from build123d import *

# Parameters (mm, degrees)
F0_R     = 1.5875
F1_DEPTH = 19.05
F0_R_2   = 3.175
F2_DEPTH = 6.35
F3_R     = 1.27


with BuildPart() as f1:
    # F0 (on Top) → F1 (new body)
    with BuildSketch(Plane.XY):
        with BuildLine():
            ThreePointArc((82.8215071839, 56.5294814298), (0, 37.38), (-82.8215071839, 56.5294814298))
            ThreePointArc((-82.8215071839, 56.5294814298), (-92.8246316261, 54.4975844509), (-93.4439756283, 44.3089870526))
            ThreePointArc((-93.4439756283, 44.3089870526), (-79.88, 0), (-93.4439756283, -44.3089870526))
            ThreePointArc((-93.4439756283, -44.3089870526), (-92.8246316261, -54.4975844509), (-82.8215071839, -56.5294814298))
            ThreePointArc((-82.8215071839, -56.5294814298), (0, -37.38), (82.8215071839, -56.5294814298))
            ThreePointArc((82.8215071839, -56.5294814298), (92.8246316261, -54.4975844509), (93.4439756283, -44.3089870526))
            ThreePointArc((93.4439756283, -44.3089870526), (79.88, 0), (93.4439756283, 44.3089870526))
            ThreePointArc((93.4439756283, 44.3089870526), (92.8246316261, 54.4975844509), (82.8215071839, 56.5294814298))
        make_face()
        with Locations((-86.5, -49)):
            Circle(F0_R, mode=Mode.SUBTRACT)
        with BuildLine():
            ThreePointArc((-44.7490329893, -12.754), (-43.0382407412, -13.2414304642), (-41.8412453259, -14.557333405))
            ThreePointArc((-41.8412453259, -14.557333405), (-39.2272080278, -18.9335940639), (-35.965811948, -22.8512647956))
            ThreePointArc((-35.965811948, -22.8512647956), (-35.1953196756, -26.0911928639), (-37.6837042763, -28.304501317))
            ThreePointArc((-37.6837042763, -28.304501317), (-53.5961461859, -32.0117479156), (-69.1555424288, -36.9971940769))
            ThreePointArc((-69.1555424288, -36.9971940769), (-72.5826288572, -36.2271539786), (-73.3024493232, -32.7891688656))
            ThreePointArc((-73.3024493232, -32.7891688656), (-70.5039949655, -24.2377869494), (-68.556245082, -15.4534970032))
            ThreePointArc((-68.556245082, -15.4534970032), (-67.4497325668, -13.5190259244), (-65.356580963, -12.754))
            Line((-65.356580963, -12.754), (-44.7490329893, -12.754))
        make_face(mode=Mode.SUBTRACT)
        with Locations((86.5, -49)):
            Circle(F0_R, mode=Mode.SUBTRACT)
        with BuildLine():
            ThreePointArc((-12.5, -12.5), (-25, 0), (-12.5, 12.5))
            Line((-12.5, 12.5), (12.5, 12.5))
            ThreePointArc((12.5, 12.5), (25, 0), (12.5, -12.5))
            Line((12.5, -12.5), (-12.5, -12.5))
        make_face(mode=Mode.SUBTRACT)
        with BuildLine():
            ThreePointArc((65.356580963, -12.754), (67.4497325668, -13.5190259244), (68.556245082, -15.4534970032))
            ThreePointArc((68.556245082, -15.4534970032), (70.5039949655, -24.2377869494), (73.3024493232, -32.7891688656))
            ThreePointArc((73.3024493232, -32.7891688656), (72.5826288572, -36.2271539786), (69.1555424288, -36.9971940769))
            ThreePointArc((69.1555424288, -36.9971940769), (53.5961461859, -32.0117479156), (37.6837042763, -28.304501317))
            ThreePointArc((37.6837042763, -28.304501317), (35.1953196756, -26.0911928639), (35.965811948, -22.8512647956))
            ThreePointArc((35.965811948, -22.8512647956), (39.2272080278, -18.9335940639), (41.8412453259, -14.557333405))
            ThreePointArc((41.8412453259, -14.557333405), (43.0382407412, -13.2414304642), (44.7490329893, -12.754))
            Line((44.7490329893, -12.754), (65.356580963, -12.754))
        make_face(mode=Mode.SUBTRACT)
        with BuildLine():
            ThreePointArc((-73.3024493232, 32.7891688656), (-72.5826288572, 36.2271539786), (-69.1555424288, 36.9971940769))
            ThreePointArc((-69.1555424288, 36.9971940769), (-53.5961461859, 32.0117479156), (-37.6837042763, 28.304501317))
            ThreePointArc((-37.6837042763, 28.304501317), (-35.1953196756, 26.0911928639), (-35.965811948, 22.8512647956))
            ThreePointArc((-35.965811948, 22.8512647956), (-39.2272080278, 18.9335940639), (-41.8412453259, 14.557333405))
            ThreePointArc((-41.8412453259, 14.557333405), (-43.0382407412, 13.2414304642), (-44.7490329893, 12.754))
            Line((-44.7490329893, 12.754), (-65.356580963, 12.754))
            ThreePointArc((-65.356580963, 12.754), (-67.4497325668, 13.5190259244), (-68.556245082, 15.4534970032))
            ThreePointArc((-68.556245082, 15.4534970032), (-70.5039949655, 24.2377869494), (-73.3024493232, 32.7891688656))
        make_face(mode=Mode.SUBTRACT)
        with Locations((-86.5, 49)):
            Circle(F0_R, mode=Mode.SUBTRACT)
        with BuildLine():
            ThreePointArc((35.965811948, 22.8512647956), (35.1953196756, 26.0911928639), (37.6837042763, 28.304501317))
            ThreePointArc((37.6837042763, 28.304501317), (53.5961461859, 32.0117479156), (69.1555424288, 36.9971940769))
            ThreePointArc((69.1555424288, 36.9971940769), (72.5826288572, 36.2271539786), (73.3024493232, 32.7891688656))
            ThreePointArc((73.3024493232, 32.7891688656), (70.5039949655, 24.2377869494), (68.556245082, 15.4534970032))
            ThreePointArc((68.556245082, 15.4534970032), (67.4497325668, 13.5190259244), (65.356580963, 12.754))
            Line((65.356580963, 12.754), (44.7490329893, 12.754))
            ThreePointArc((44.7490329893, 12.754), (43.0382407412, 13.2414304642), (41.8412453259, 14.557333405))
            ThreePointArc((41.8412453259, 14.557333405), (39.2272080278, 18.9335940639), (35.965811948, 22.8512647956))
        make_face(mode=Mode.SUBTRACT)
        with Locations((86.5, 49)):
            Circle(F0_R, mode=Mode.SUBTRACT)
    extrude(amount=F1_DEPTH)

    # F0 (on Top) → F2 (cut)
    with BuildSketch(Plane.XY):
        with BuildLine():
            Line((12.5, 12.5), (-12.5, 12.5))
            ThreePointArc((-12.5, 12.5), (-25, 0), (-12.5, -12.5))
            Line((-12.5, -12.5), (12.5, -12.5))
            ThreePointArc((12.5, -12.5), (25, 0), (12.5, 12.5))
        make_face()
        with Locations((-12.5, 0)):
            Circle(F0_R_2, mode=Mode.SUBTRACT)
        with Locations((12.5, 0)):
            Circle(F0_R_2, mode=Mode.SUBTRACT)
    extrude(amount=F2_DEPTH, mode=Mode.SUBTRACT)

    # F3
    f3_edges = [f1.edges().sort_by_distance(p)[0] for p in [
        (-79.88, 0, 19.05),
        (-92.824632, -54.497584, 19.05),
        (0, -37.38, 19.05),
        (92.824632, -54.497584, 19.05),
        (79.88, 0, 19.05),
        (92.824632, 54.497584, 19.05),
        (0, 37.38, 19.05),
        (-92.824632, 54.497584, 19.05),
    ]]
    fillet(f3_edges, radius=F3_R)


solid = f1.part
Here's how the part is built. I have some questions about the finished solid (model axes, mm). A direction names the side the tool comes from. Coordinates: 2 decimals unless noted, no trailing zeros. Write each loop counter-clockwise with the first axis right and the second up, starting at its lowest first coordinate (ties: lowest second). Pieces come first, ordered by that corner, then holes.
1) If we section it at B-B (z = 9.5): Count the separate pieces of the cut face and the enclosed holes in it, plus the area to 3 significant figures.
Filled in:
separate pieces: 1
enclosed holes: 9
area: 11,600 mm2
2) If I drill on line 1 (Y direction, x = 86.5, z = 10.5); line 2 (X direction, y = -21.5, z = 9.25); line 3 (X direction, y = -23, z = 9), over which ranges is the centre line in solid material (lowest first)?
Filled in:
line 1: y = -57.38 to -50.59, -47.41 to -31.69, 31.69 to 47.41, 50.59 to 57.38
line 2: x = -82.86 to -69.8, -37.21 to 37.21, 69.8 to 82.86
line 3: x = -83.3 to -70.17, -35.83 to 35.83, 70.17 to 83.3
3) I'm going to push flat-ended pins straight in: pin 1 (5.5 mm diameter, centred on x = 4, z = 12.5, fed in from -Y); pin 2 (1.5 mm diameter, centred on x = 38, z = 10.5, fed in from +Y); pin 3 (9.5 mm diameter, centred on x = -50.5, z = 6.5, fed in from -Y). Where does each tip first touch, or does it pass through?
Filled in:
pin 1: stops at y = -37.5
pin 2: stops at y = 41.4
pin 3: stops at y = -45.65
4) Which directions (+Z, -Z, +X, -X, +Y, -Y) give clear straight access to the entire face, cutting with the end or side of a thin tool? Please do faces 3 (the face through (79.883, -0.658, 8.766)), 4 (the face through (53.817, -32.073, 9.392)).
Filled in:
face 3: +Z, -Z, +X
face 4: +Z, -Z
5) If we section it at A-A (y = 0): List the corners of the cut face in (x, z) for me, plus the area to 3 significant figures.
Filled in:
outline: (-79.88, 0) - (-25, 0) - (-25, 19.05) - (-78.61, 19.05) arc R1.27 ccw to (-79.88, 17.78) - close; (25, 0) - (79.88, 0) - (79.88, 17.78) arc R1.27 ccw to (78.61, 19.05) - (25, 19.05) - close
area: 2,090 mm2
6) Thinking about a two-plate mould opening in Y: for faces 1 (the face through (-1, 14, 0)), 2 (the face through (55, -12.754, 9)), which applies, +Y half, -Y half, draft (parallel to the pull), parting line (faces both ways), or undercut?
Filled in:
face 1: draft
face 2: undercut
